Part print with two shaded views. Sizes in mm from the minimum x, y, z corner. A direction names the side the tool comes from. Round coordinates to 2 decimals unless told otherwise and drop trailing zeros. Order: outer loops, then holes, each group sorted by start corner. A loop starts at its lowest first (then second) coordinate and runs counter-clockwise, first axis right, second up. Notation, with made-up numbers: (20, 19.25) - (43, 19.25) arc R15 ccw to (43, 24.25) - close; hole circle Ø8 at (42.25, 43.5). An arc over 180 degrees is marked (long way). Write item = value, one per line.
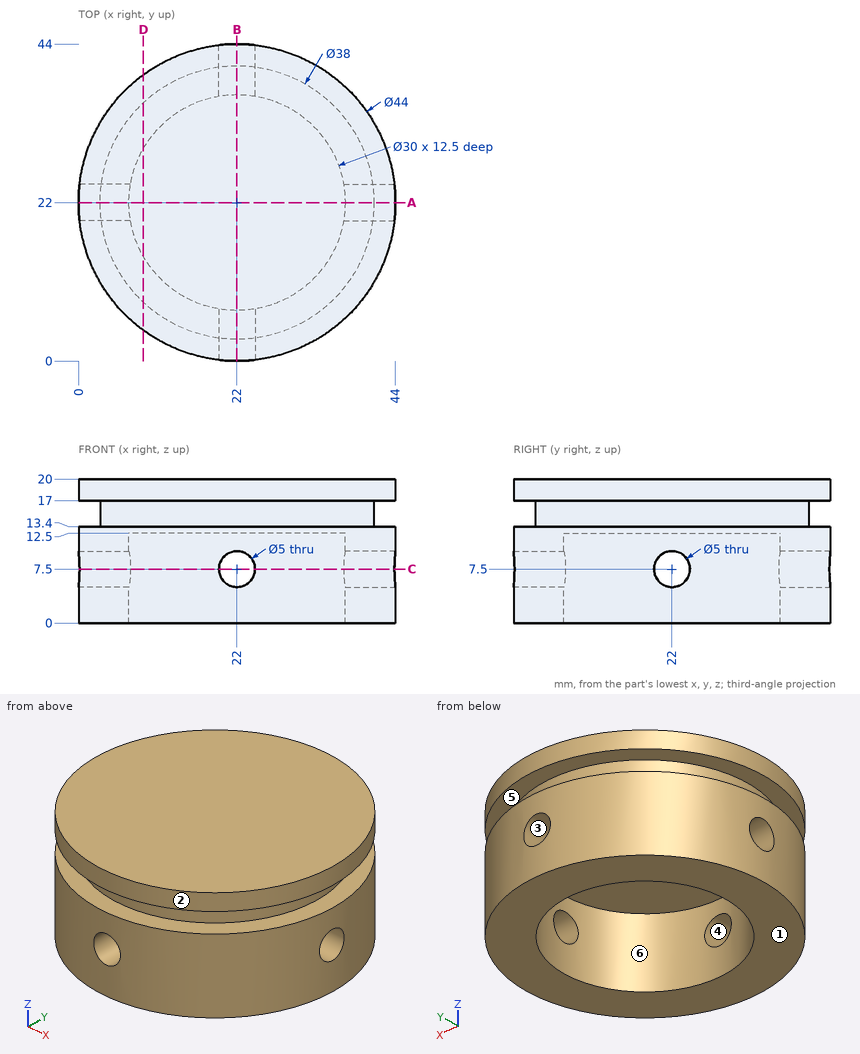
1) Cut at A-A (y = 22). Write the cut outline in (x, z).
Conclusion:
outline = (0, 0) - (7, 0) - (7, 5) - (0, 5) - close; (0, 10) - (7, 10) - (7, 12.5) - (37, 12.5) - (37, 10) - (44, 10) - (44, 13.4) - (41, 13.4) - (41, 17) - (44, 17) - (44, 20) - (0, 20) - (0, 17) - (3, 17) - (3, 13.4) - (0, 13.4) - close; (37, 0) - (44, 0) - (44, 5) - (37, 5) - close
2) Mould opens along X. For the marked faces 1, 2 and 3 say: +X half, -X half, draft (parallel to the pull), parting line (faces both ways), or undercut.
Conclusion:
face_1 = draft
face_2 = parting line
face_3 = undercut
3) 3-axis set-ups, long thin cutter, end or side, ignore diameter. For the marked faces 4, 5 and 6: which of +Z, -Z, +X, -X, +Y, -Y reach the whole face in a straight line?
Conclusion:
face_4 = +Y, -Y
face_5 = none
face_6 = -Z
4) Flat gauge pins, fed straight in: pin 1 Ø1.5 at (y, z) = (35.5, 8.5) entering from +X; pin 2 Ø4 at (y, z) = (22, 7.5) entering from +X; pin 3 Ø12 at (x, z) = (7, 8.5) entering from +Y; pin 4 Ø1.5 at (y, z) = (7.5, 7) entering from -X. Where does each tip first touch, or does it go through?
Conclusion:
pin_1 = 39.93
pin_2 = through
pin_3 = 42.07
pin_4 = 4.83
5) Cut at D-D (x = 9). Write the cut outline in (y, z).
Conclusion:
outline = (4.25, 0) - (14.52, 0) - (14.52, 12.5) - (29.48, 12.5) - (29.48, 0) - (39.75, 0) - (39.75, 13.4) - (35.86, 13.4) - (35.86, 17) - (39.75, 17) - (39.75, 20) - (4.25, 20) - (4.25, 17) - (8.14, 17) - (8.14, 13.4) - (4.25, 13.4) - close
6) Cut at C-C (z = 7.5). Write the cut outline in (x, y), and give its area (3 significant figures).
Conclusion:
outline = (0.14, 19.5) arc R22 ccw to (19.5, 0.14) - (19.5, 7.21) arc R15 cw to (7.21, 19.5) - close; (0.14, 24.5) - (7.21, 24.5) arc R15 cw to (19.5, 36.79) - (19.5, 43.86) arc R22 ccw to start; (24.5, 0.14) arc R22 ccw to (43.86, 19.5) - (36.79, 19.5) arc R15 cw to (24.5, 7.21) - close; (24.5, 36.79) arc R15 cw to (36.79, 24.5) - (43.86, 24.5) arc R22 ccw to (24.5, 43.86) - close
area = 673 mm^2
7) Wall check: line 1 along Z through (x, y) = (21.5, 27.5); line 2 along X through (y, z) = (34, 10); line 3 along Y through (x, z) = (15, 12). Give the ranges that are in metal, low to high.
Conclusion:
line_1 = 12.5 to 20
line_2 = 3.56 to 13, 31 to 40.44
line_3 = 1.14 to 8.73, 35.27 to 42.86
